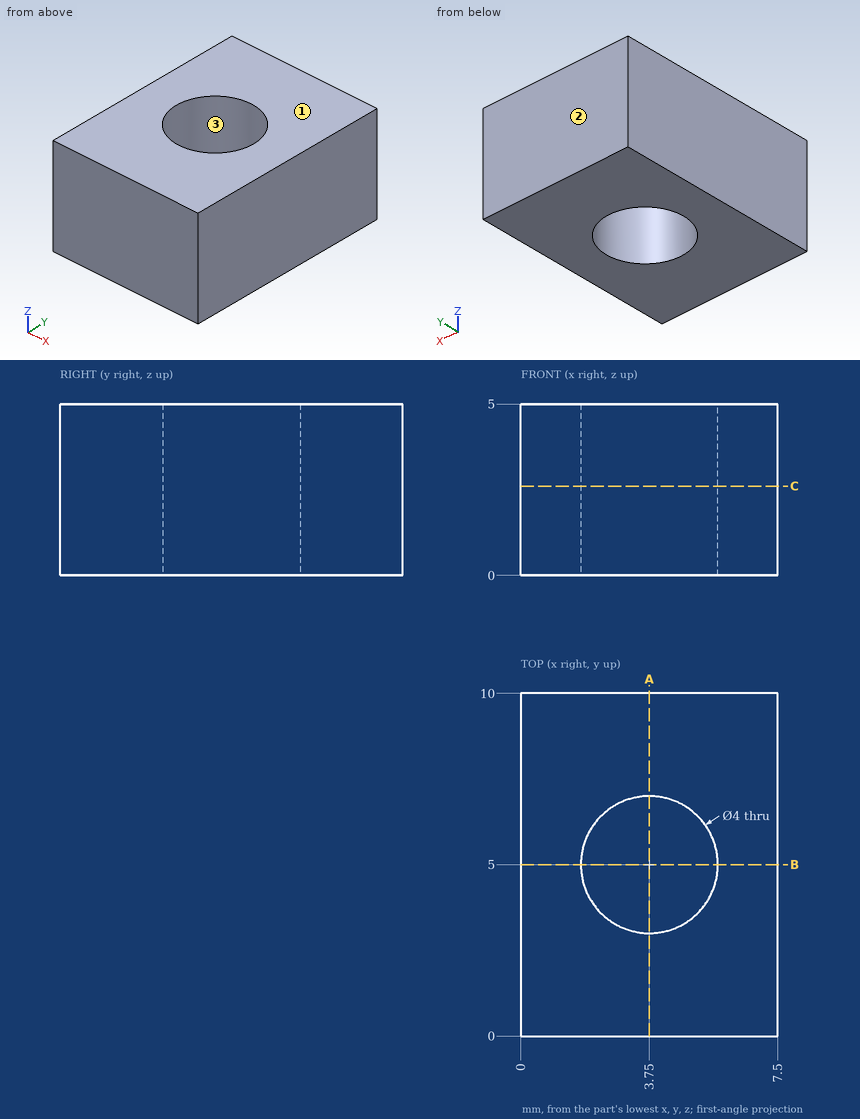
Verification items for this drawing (mm, ordinates from the low corner). Coordinates: 2 decimals unless noted, no trailing zeros. Loops run counter-clockwise (first coordinate to the right, second up) from the corner with the lowest first, then second, coordinate; pieces in that order, holes last. Notation, with made-up numbers: (70.25, -2) - (123.25, -2) arc R22 cw to (123.25, 4) - close; hole circle Ø5 at (31.5, 75.5). An arc over 180 degrees is marked (long way). One line per item, written item: value. Start each with the question number.
(1) Depth check by flat-ended pin: P1, Ø3, axis at x = 3.75, y = 5, coming from the +Z side. Enter the tip coordinate at first touch or a pass-through.
(2) Material ranges on line 1 (Y direction, x = 3.75, z = 2.85); line 2 (X direction, y = 4.25, z = 2.2); line 3 (Y direction, x = 5.5, z = 2.95), recorded low to high. Write a range as [from, to].
(3) Mould release check, pull along Y, two halves, no side actions. Record for the marked faces 1, 2 and 3: released by +Y, released by -Y, zero draft, split by the parting line, or undercut.
(4) Cross-section at A-A on x = 3.75. Enter the section's corners in (y, z), plus the area to 3 significant figures.
(5) Cross-section at C-C on z = 2.6. Enter the section's corners in (x, y), plus the area to 3 significant figures.
(6) Cross-section at B-B on y = 5. Enter the section's corners in (x, z).
Results below:
1. P1: passes through
2. line 1: y = [0, 3], [7, 10]
2. line 2: x = [0, 1.9], [5.6, 7.5]
2. line 3: y = [0, 4.03], [5.97, 10]
3. face 1: zero draft
3. face 2: released by +Y
3. face 3: undercut
4. outline: (0, 0) - (3, 0) - (3, 5) - (0, 5) - close; (7, 0) - (10, 0) - (10, 5) - (7, 5) - close
4. area: 30.0 mm2
5. outline: (0, 0) - (7.5, 0) - (7.5, 10) - (0, 10) - close; hole circle Ø4 at (3.75, 5)
5. area: 62.4 mm2
6. outline: (0, 0) - (1.75, 0) - (1.75, 5) - (0, 5) - close; (5.75, 0) - (7.5, 0) - (7.5, 5) - (5.75, 5) - close
